Geometry check sheet. Reference: the model listing, model coordinates, mm. A direction names the side the tool comes from. Round coordinates to 2 decimals unless told otherwise and drop trailing zeros. Order: outer loops, then holes, each group sorted by start corner. A loop starts at its lowest first (then second) coordinate and runs counter-clockwise, first axis right, second up.
(1) Go/stop test with flat-tipped pins: pin 1 (1.5 mm diameter, centred on x = -4.5, y = -12, fed in from -Z); pin 2 (3 mm diameter, centred on y = 0, z = 26.035, fed in from -X); pin 3 (5 mm diameter, centred on x = 0.5, y = 1.5, fed in from +Z) (3 decimals); pin 4 (4 mm diameter, centred on x = -17, z = 14.5, fed in from -Y). Record where each tip stops, or that it passes through.
(2) Sectioned sample at B-B (y = 0). Give the number of separate pieces and of enclosed holes in the cut face, plus the area to 3 significant figures.
(3) Set-up check for faces 1 (the face through (18.17, 5.72, 16.95)), 2 (the face through (4, 19, 31.115)), 3 (the face through (-0.221, 9.687, 1.565)), 4 (the face through (21.199, 6.676, 15.697)), 5 (the face through (-20.58, 0.48, 19.44)): record each of +Z, -Z, +X, -X, +Y, -Y from which the full face is reachable in a straight line by a thin tool's end or side.
(4) Sectioned sample at A-A (x = 0). Record the boundary of the cut face in (y, z) (3 decimals), plus the area to 3 significant figures.
(5) Material ranges on line 1 along Z through (x, y) = (15, 19.5) (3 decimals); line 2 along Y through (x, z) = (0, 1.1); line 3 along X through (y, z) = (0, 16.5) (3 decimals), recorded low to high.
(6) Release check for a two-part mould opening along Z. For faces 6 (the face through (0, 0, 0)), 7 (the face through (-0.1, -22.5, 28.575)), 8 (the face through (0, 0, 3.175)) record: +Z half, -Z half, draft (parallel to the pull), parting line (faces both ways), or undercut.
(7) Sectioned sample at C-C (y = 7). Record the boundary of the cut face in (x, z) (3 decimals), plus the area to 3 significant figures.
(8) Sectioned sample at D-D (z = 14). Record the boundary of the cut face in (x, y) (3 decimals), plus the area to 3 significant figures.
from build123d import *

# Parameters (mm, degrees)
SKETCH1_R           = 25.4
SKETCH1_R_2         = 1.7
BOSS_EXTRUDE1_DEPTH = 3.175
SKETCH4_R           = 22.225
SKETCH4_R_2         = 19.05
BOSS_EXTRUDE2_DEPTH = 25.4
SKETCH5_R           = 25.4
SKETCH5_R_2         = 19.05
BOSS_EXTRUDE3_DEPTH = 2.54
SKETCH6_R           = 1.5875
CUT_EXTRUDE1_DEPTH  = 26.4


with BuildPart() as part:
    # Sketch1 → Boss-Extrude1 (new body)
    with BuildSketch(Plane.XY):
        Circle(SKETCH1_R)
        with Locations((0, -8.001)):
            Circle(SKETCH1_R_2, mode=Mode.SUBTRACT)
        with Locations((0, 8.001)):
            Circle(SKETCH1_R_2, mode=Mode.SUBTRACT)
        with Locations((-6.929069256, 4.0005)):
            Circle(SKETCH1_R_2, mode=Mode.SUBTRACT)
        with Locations((-6.929069256, -4.0005)):
            Circle(SKETCH1_R_2, mode=Mode.SUBTRACT)
        with Locations((6.929069256, -4.0005)):
            Circle(SKETCH1_R_2, mode=Mode.SUBTRACT)
        with Locations((6.929069256, 4.0005)):
            Circle(SKETCH1_R_2, mode=Mode.SUBTRACT)
    extrude(amount=BOSS_EXTRUDE1_DEPTH)

    # Sketch4 → Boss-Extrude2 (add)
    with BuildSketch(Plane.XY.offset(3.175)):
        Circle(SKETCH4_R)
        Circle(SKETCH4_R_2, mode=Mode.SUBTRACT)
    extrude(amount=BOSS_EXTRUDE2_DEPTH)

    # Sketch5 → Boss-Extrude3 (add)
    with BuildSketch(Plane.XY.offset(28.575)):
        Circle(SKETCH5_R)
        Circle(SKETCH5_R_2, mode=Mode.SUBTRACT)
    extrude(amount=BOSS_EXTRUDE3_DEPTH)

    # Sketch6 → Cut-Extrude1 (cut, through all)
    with BuildSketch(Plane(origin=(0, 0, 0), x_dir=(0, 0, -1), z_dir=(1, 0, 0))):
        with Locations((-26.035, 0)):
            Circle(SKETCH6_R)
        with Locations((-20.955, 0)):
            Circle(SKETCH6_R)
    extrude(amount=-CUT_EXTRUDE1_DEPTH, mode=Mode.SUBTRACT)


solid = part.part
Answer below:
1. pin 1: stops at z = 0
1. pin 2: stops at x = 18.99
1. pin 3: stops at z = 3.175
1. pin 4: stops at y = -16.4
2. separate pieces: 3
2. enclosed holes: 0
2. area: 335 mm2
3. face 1: +Z
3. face 2: +Z, +X, -X, +Y, -Y
3. face 3: +Z, -Z
3. face 4: none
3. face 5: -X
4. outline: (-25.4, 0) - (-9.701, 0) - (-9.701, 3.175) - (-19.05, 3.175) - (-19.05, 31.115) - (-25.4, 31.115) - (-25.4, 28.575) - (-22.225, 28.575) - (-22.225, 3.175) - (-25.4, 3.175) - close; (-6.301, 0) - (6.301, 0) - (6.301, 3.175) - (-6.301, 3.175) - close; (9.701, 0) - (25.4, 0) - (25.4, 3.175) - (22.225, 3.175) - (22.225, 28.575) - (25.4, 28.575) - (25.4, 31.115) - (19.05, 31.115) - (19.05, 3.175) - (9.701, 3.175) - close
4. area: 333 mm2
5. line 1: z = 0 to 3.175, 28.575 to 31.115
5. line 2: y = -25.4 to -9.7, -6.3 to 6.3, 9.7 to 25.4
5. line 3: x = -22.225 to -19.05, 19.05 to 22.225
6. face 6: -Z half
6. face 7: undercut
6. face 8: +Z half
7. outline: (-24.416, 0) - (-1.374, 0) - (-1.374, 3.175) - (-17.717, 3.175) - (-17.717, 31.115) - (-24.416, 31.115) - (-24.416, 28.575) - (-21.094, 28.575) - (-21.094, 3.175) - (-24.416, 3.175) - close; (1.374, 0) - (24.416, 0) - (24.416, 3.175) - (21.094, 3.175) - (21.094, 28.575) - (24.416, 28.575) - (24.416, 31.115) - (17.717, 31.115) - (17.717, 3.175) - (1.374, 3.175) - close
7. area: 352 mm2
8. outline: circle Ø44.45 at (0, 0); hole circle Ø38.1 at (0, 0)
8. area: 412 mm2
